Autodesk Inventor part; units mm, degrees
ref_plane "YZ Plane" through (0, 0, 0) normal (1, 0, 0) x (0, 1, 0)
ref_plane "XZ Plane" through (0, 0, 0) normal (0, 1, 0) x (-1, 0, 0)
ref_plane "XY Plane" through (0, 0, 0) normal (0, 0, 1) x (1, 0, 0)
sketch "Sketch1" plane through (0, 0, 0) normal (1, 0, 0) x (0, 1, 0)
  circle A0 centre (0, 0) radius 7.5
  circle A1 centre (0, 0) radius 9
  circle A2 centre (0, 0) radius 15
  dimension "d0" = 15
  dimension "d1" = 18
  dimension "d2" = 30
extrude "Extrusion1" add sketch "Sketch1" against normal blind 5 contours A1 | A2
extrude "Extrusion2" add sketch "Sketch1" along normal blind 10 contours A1
sketch "Sketch2" plane through (0, 0, 0) normal (1, 0, 0) x (0, 0, -1)
  point P0 (0, 0)
  point P1 (12, 0)
  dimension "d7" = 12
hole "Hole1" at (0, 0, -12) direction (-1, 0, 0) diameter 3 end through all counterbore diameter 4 counterbore depth 2
pattern_circular "Circular Pattern1" count 5 over 360 about axis through (0, 0, 0) along (-1, 0, 0) of "Hole1"
Model file for the job. Use its own axes, mm. A direction names the side the tool comes from. Coordinates: 2 decimals unless noted, no trailing zeros. Loops run counter-clockwise (first coordinate to the right, second up) from the corner with the lowest first, then second, coordinate; pieces in that order, holes last. Notation, with made-up numbers: (7, 80) - (63, 80) arc R26 ccw to (63, 108) - close; hole circle Ø3 at (84.25, 70.25). An arc over 180 degrees is marked (long way). Write item = value, one per line. Start each with the question number.
Item 1: 3-axis set-ups, long thin cutter, end or side, ignore diameter. For faces 1 (the face through (-3.521, -8.537, 9.486)), 2 (the face through (-1, 1.2, -10.4)): which of +Z, -Z, +X, -X, +Y, -Y reach the whole face in a straight line?
Item 2: Drop flat-ended pins along their axis: pin 1 Ø3 at (y, z) = (4, 3) entering from -X; pin 2 Ø5 at (y, z) = (11.41, -3.71) entering from +X; pin 3 Ø3 at (x, y) = (0.5, -3.5) entering from -Z; pin 4 Ø3.5 at (y, z) = (-7.05, 9.71) entering from +X. Give the stop position or say it passes through.
Item 3: Saw through at D-D, the plane z = -3. List the corners of the cut face in (x, y), then the cut area to 3 significant figures.
Item 4: Saw through at C-C, the plane x = 3.25. List the corners of the cut face in (y, z), then the cut area to 3 significant figures.
Item 5: Saw through at B-B, the plane y = 0. List the corners of the cut face in (x, z), then the cut area to 3 significant figures.
Item 6: Saw through at A-A, the plane z = -12. List the corners of the cut face in (x, y).
Item 7: Wall check: probe 1 along X at (y, z) = (11.25, 5.25); probe 2 along Z at (x, y) = (1, -1); probe 3 along Y at (x, z) = (-2.5, 3.5). Give the ranges that are in metal, low to high. Write a range as [from, to].
Item 8: Pull direction Z, two halves, no side cores. Call faces 3 (the face through (0, 6.5, -6.5)), 4 (the face through (2.395, -7.493, -0.33)), 5 (the face through (4.93, -1.172, -8.923)): +Z half, -Z half, draft (parallel to the pull), parting line (faces both ways), or undercut.
Answers:
q1.face_1 = +X, -X
q1.face_2 = +X
q2.pin_1 = through
q2.pin_2 = 0
q2.pin_3 = -14.85
q2.pin_4 = -2
q3.outline = (-5, -14.7) - (0, -14.7) - (0, -13.28) - (-2, -13.28) - (-2, -12.73) - (-5, -12.73) - close; (-5, -10.09) - (-2, -10.09) - (-2, -9.54) - (0, -9.54) - (0, -8.49) - (10, -8.49) - (10, -6.87) - (-5, -6.87) - close; (-5, 6.87) - (10, 6.87) - (10, 8.49) - (0, 8.49) - (0, 9.54) - (-2, 9.54) - (-2, 10.09) - (-5, 10.09) - close; (-5, 12.73) - (-2, 12.73) - (-2, 13.28) - (0, 13.28) - (0, 14.7) - (-5, 14.7) - close
q3.area = 79.6 mm2
q4.outline = circle Ø18 at (0, 0); hole circle Ø15 at (0, 0)
q4.area = 77.8 mm2
q5.outline = (-5, -15) - (0, -15) - (0, -14) - (-2, -14) - (-2, -13.5) - (-5, -13.5) - close; (-5, -10.5) - (-2, -10.5) - (-2, -10) - (0, -10) - (0, -9) - (10, -9) - (10, -7.5) - (-5, -7.5) - close; (-5, 7.5) - (10, 7.5) - (10, 9) - (0, 9) - (0, 15) - (-5, 15) - close
q5.area = 88.0 mm2
q6.outline = (-5, -9) - (0, -9) - (0, -2) - (-2, -2) - (-2, -1.5) - (-5, -1.5) - close; (-5, 1.5) - (-2, 1.5) - (-2, 2) - (0, 2) - (0, 9) - (-5, 9) - close
q7.probe_1 = [-5, 0]
q7.probe_2 = [-8.94, -7.43], [7.43, 8.94]
q7.probe_3 = [-14.59, -6.63], [6.63, 14.59]
q8.face_3 = draft
q8.face_4 = undercut
q8.face_5 = parting line
